Here's how the part is built. I have some questions about the finished solid (model axes, mm). Coordinates: 2 decimals unless noted, no trailing zeros. Loops run counter-clockwise (first coordinate to the right, second up) from the corner with the lowest first, then second, coordinate; pieces in that order, holes last.
from build123d import *

# Parameters (mm, degrees)
SKETCH_1_R      = 1.5
EXTRUDE_1_DEPTH = 3


with BuildPart() as part:
    # 草图1 → 凸台-拉伸1 (new body)
    with BuildSketch(Plane.XY):
        with BuildLine():
            Line((0, 0), (40, 0))
            Line((40, 0), (40, -17))
            Line((40, -17), (38, -17))
            Line((38, -17), (38, -13))
            ThreePointArc((38, -13), (35.000000014, -10.000000014), (32.000000029, -13))
            Line((32.000000029, -13), (32.000000029, -17))
            ThreePointArc((32.000000029, -17), (32.878679681, -19.121320333), (35.000000014, -20))
            Line((35.000000014, -20), (43.000000014, -20))
            ThreePointArc((43.000000014, -20), (45.121320358, -19.121320344), (46.000000014, -17))
            Line((46.000000014, -17), (46.000000014, 0))
            Line((46.000000014, 0), (69.5, 0))
            Line((69.5, 0), (69.5, -7))
            Line((69.5, -7), (72.5, -7))
            Line((72.5, -7), (72.5, 0))
            Line((72.5, 0), (75.5, 0))
            Line((75.5, 0), (75.5, -23))
            Line((75.5, -23), (72.5, -23))
            Line((72.5, -23), (72.5, -16))
            Line((72.5, -16), (69.5, -16))
            Line((69.5, -16), (69.5, -65.5))
            Line((69.5, -65.5), (72.5, -65.5))
            Line((72.5, -65.5), (72.5, -58.5))
            Line((72.5, -58.5), (75.5, -58.5))
            Line((75.5, -58.5), (75.5, -81.5))
            Line((75.5, -81.5), (72.5, -81.5))
            Line((72.5, -81.5), (72.5, -74.5))
            Line((72.5, -74.5), (69.5, -74.5))
            Line((69.5, -74.5), (69.5, -86))
            Line((69.5, -86), (0, -86))
            Line((0, -86), (0, -74.5))
            Line((0, -74.5), (-3, -74.5))
            Line((-3, -74.5), (-3, -81.5))
            Line((-3, -81.5), (-6, -81.5))
            Line((-6, -81.5), (-6, -58.5))
            Line((-6, -58.5), (-3, -58.5))
            Line((-3, -58.5), (-3, -65.5))
            Line((-3, -65.5), (0, -65.5))
            Line((0, -65.5), (0, -16))
            Line((0, -16), (-3, -16))
            Line((-3, -16), (-3, -23))
            Line((-3, -23), (-6, -23))
            Line((-6, -23), (-6, 0))
            Line((-6, 0), (-3, 0))
            Line((-3, 0), (-3, -7))
            Line((-3, -7), (0, -7))
            Line((0, -7), (0, 0))
        make_face()
        with Locations((15, -67)):
            Circle(SKETCH_1_R, mode=Mode.SUBTRACT)
        with Locations((44, -67)):
            Circle(SKETCH_1_R, mode=Mode.SUBTRACT)
        with Locations((15, -35)):
            Circle(SKETCH_1_R, mode=Mode.SUBTRACT)
        with Locations((44, -35)):
            Circle(SKETCH_1_R, mode=Mode.SUBTRACT)
        with Locations((-1.5, -70)):
            Circle(SKETCH_1_R, mode=Mode.SUBTRACT)
        with Locations((70.793087485, -70)):
            Circle(SKETCH_1_R, mode=Mode.SUBTRACT)
        with Locations((-1.5, -11.5)):
            Circle(SKETCH_1_R, mode=Mode.SUBTRACT)
        with Locations((70.793087485, -11.5)):
            Circle(SKETCH_1_R, mode=Mode.SUBTRACT)
    extrude(amount=EXTRUDE_1_DEPTH)


solid = part.part
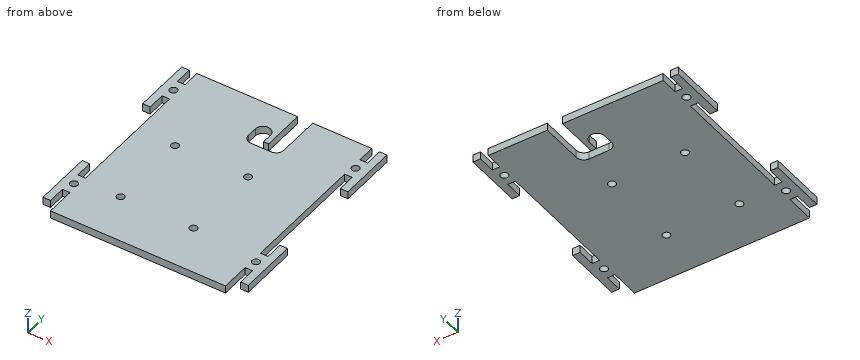
Q1. Please list where these lines run through material, in increasing order: probe 1 along X at (y, z) = (-61, 2.6); probe 2 along X at (y, z) = (-70, 1.1); probe 3 along X at (y, z) = (-16.5, 1.6).
Q2. Suppose I cut it at B-B on x = -1.5. Write out the boundary of the cut face in (y, z).
Q3. Will these pins go through, and if not, where does the flat tip stop? P1, Ø0.9, axis at x = -4.5, z = 2, coming from the -Y side; P2, Ø0.9, axis at x = 70.5, z = 1.5, coming from the +Y side; P3, Ø1.5, axis at x = -1, z = 1, coming from the -Y side.
Q4. Suppose I cut it at C-C on x = 44. Write out the boundary of the cut face in (y, z), and give its area (3 significant figures).
Q5. Suppose I cut it at A-A on y = -35. Write out the boundary of the cut face in (x, z).
Q6. Suppose I cut it at D-D on y = -11.5. Write out the boundary of the cut face in (x, z), and give its area (3 significant figures).
Check values:
1. probe 1: x = -6 to -3, 0 to 69.5, 72.5 to 75.5
1. probe 2: x = -6 to -3, 0 to 69.29, 72.29 to 75.5
1. probe 3: x = -6 to -3, 0 to 32, 38 to 40, 46 to 69.5, 72.5 to 75.5
2. outline: (-74.5, 0) - (-71.5, 0) - (-71.5, 3) - (-74.5, 3) - close; (-68.5, 0) - (-65.5, 0) - (-65.5, 3) - (-68.5, 3) - close; (-16, 0) - (-13, 0) - (-13, 3) - (-16, 3) - close; (-10, 0) - (-7, 0) - (-7, 3) - (-10, 3) - close
3. P1: stops at y = -81.5
3. P2: stops at y = -7
3. P3: stops at y = -74.5
4. outline: (-86, 0) - (-68.5, 0) - (-68.5, 3) - (-86, 3) - close; (-65.5, 0) - (-36.5, 0) - (-36.5, 3) - (-65.5, 3) - close; (-33.5, 0) - (-19.83, 0) - (-19.83, 3) - (-33.5, 3) - close
4. area: 181 mm2
5. outline: (0, 0) - (13.5, 0) - (13.5, 3) - (0, 3) - close; (16.5, 0) - (42.5, 0) - (42.5, 3) - (16.5, 3) - close; (45.5, 0) - (69.5, 0) - (69.5, 3) - (45.5, 3) - close
6. outline: (-6, 0) - (-3, 0) - (-3, 3) - (-6, 3) - close; (0, 0) - (32.4, 0) - (32.4, 3) - (0, 3) - close; (37.6, 0) - (40, 0) - (40, 3) - (37.6, 3) - close; (46, 0) - (69.29, 0) - (69.29, 3) - (46, 3) - close; (72.29, 0) - (75.5, 0) - (75.5, 3) - (72.29, 3) - close
6. area: 193 mm2
